Input: part model. Units: mm. Frame: model coordinates. A direction names the side the tool comes from. Round coordinates to 2 decimals unless told otherwise and drop trailing zeros. Loops run counter-clockwise (first coordinate to the right, second up) from the corner with the lowest first, then second, coordinate; pieces in that order, holes last. Notation, with made-up numbers: (-3.5, 69) - (13.5, 69) arc R28 ccw to (13.5, 93) - close; hole circle Ø3 at (-19, -1). An arc over 180 degrees is marked (long way). One line per question, with ' | ' between items. Start each with the question number.
Item 1: Section B-B, the plane z = 1.55. Return loops of the section in (x, y), plus the area to 3 significant figures.
Item 2: Material intervals for line 1 along X through (y, z) = (18.5, 1.85); line 2 along X through (y, z) = (35, 0.4); line 3 along X through (y, z) = (2.5, 2.4), sorted ascending.
Item 3: Section A-A, the plane y = 24.5. Return loops of the section in (x, z), plus the area to 3 significant figures.
Item 4: Section C-C, the plane x = -2.5. Return loops of the section in (y, z), plus the area to 3 significant figures.
Item 5: First-contact query: pin 1 (1.5 mm diameter, centred on x = -70.5, z = 1.5, fed in from +Y); pin 2 (0.9 mm diameter, centred on y = 17.5, z = 1, fed in from -X). Flat tips, straight axial feed; report the tip coordinate or a pass-through.
Item 6: Draft query along Y for faces 1 (the face through (7.729, 32.186, 1.521)), 2 (the face through (72.375, 19, 1)), 3 (the face through (-63.973, 35.741, 1.521)). Return one class per face: pulls with the +Y half, pulls with the -Y half, needs draft (parallel to the pull), parting line crosses it, or undercut.
Item 7: Set-up query: faces 4 (the face through (-71, -1.252, 1)), 5 (the face through (-71, 8.748, 1)), 6 (the face through (75.227, 1.755, 1.521)), 7 (the face through (86, 8.748, 1)), 8 (the face through (7, 29, 3)). Return all of +Z, -Z, +X, -X, +Y, -Y with unobstructed straight access to the full face (end or side cutting, diameter ignored); none if empty.
```python
from build123d import *

# Parameters (mm, degrees)
SKETCH2_R           = 1.6
BOSS_EXTRUDE1_DEPTH = 3
CUT_EXTRUDE1_REACH  = 100.01
SKETCH3_R           = 1.6
FILLET1_R           = 10
FILLET2_R           = 2


with BuildPart() as part:
    # Sketch2 → Boss-Extrude1 (new body)
    with BuildSketch(Plane.XY):
        Polygon((-74.424572317, -1.251944012), (-56.824572317, -1.251944012), (-56.824572317, 28.748055988), (72.375427683, 28.748055988), (72.375427683, -1.251944012), (89.975427683, -1.251944012), (89.975427683, 8.748055988), (82.375427683, 8.748055988), (82.375427683, 38.748055988), (-66.824572317, 38.748055988), (-66.824572317, 8.748055988), (-74.424572317, 8.748055988), align=None)
        with Locations((-70.424572317, 3.748055988)):
            Circle(SKETCH2_R, mode=Mode.SUBTRACT)
        with Locations(Location((85.975427683, 3.748055988, 0), (0, 0, 180))):
            Circle(SKETCH2_R, mode=Mode.SUBTRACT)
    extrude(amount=BOSS_EXTRUDE1_DEPTH)

    # Sketch3 → Cut-Extrude1 (cut, up to next)
    with BuildSketch(Plane.XY.offset(3), mode=Mode.PRIVATE) as cut_extrude1_sk1:
        with Locations((-36.924572317, 33.748055988)):
            Circle(SKETCH3_R)
    cut_extrude1_tool1 = extrude(cut_extrude1_sk1.sketch, amount=-CUT_EXTRUDE1_REACH, mode=Mode.PRIVATE) & part.part
    # Sketch3 → Cut-Extrude1 (cut, up to next)
    with BuildSketch(Plane.XY.offset(3), mode=Mode.PRIVATE) as cut_extrude1_sk2:
        with Locations((8.075427683, 33.748055988)):
            Circle(SKETCH3_R)
    cut_extrude1_tool2 = extrude(cut_extrude1_sk2.sketch, amount=-CUT_EXTRUDE1_REACH, mode=Mode.PRIVATE) & part.part
    # Sketch3 → Cut-Extrude1 (cut, up to next)
    with BuildSketch(Plane.XY.offset(3), mode=Mode.PRIVATE) as cut_extrude1_sk3:
        with Locations((53.075427683, 33.748055988)):
            Circle(SKETCH3_R)
    cut_extrude1_tool3 = extrude(cut_extrude1_sk3.sketch, amount=-CUT_EXTRUDE1_REACH, mode=Mode.PRIVATE) & part.part
    add(cut_extrude1_tool1.solids().sort_by_distance((-36.924572, 33.748056, 3))[0], mode=Mode.SUBTRACT)
    add(cut_extrude1_tool2.solids().sort_by_distance((8.075428, 33.748056, 3))[0], mode=Mode.SUBTRACT)
    add(cut_extrude1_tool3.solids().sort_by_distance((53.075428, 33.748056, 3))[0], mode=Mode.SUBTRACT)

    # Fillet1
    fillet1_edges = [part.edges().sort_by_distance(p)[0] for p in [
        (-66.824572317, 38.748055988, 1.5),
        (82.375427683, 38.748055988, 1.5),
        (72.375427683, -1.251944012, 1.5),
        (-56.824572317, -1.251944012, 1.5),
    ]]
    fillet(fillet1_edges, radius=FILLET1_R)

    # Fillet2
    fillet2_edges = [part.edges().sort_by_distance(p)[0] for p in [
        (-74.424572317, 8.748055988, 1.5),
        (-66.824572317, 8.748055988, 1.5),
        (82.375427683, 8.748055988, 1.5),
        (89.975427683, 8.748055988, 1.5),
    ]]
    fillet(fillet2_edges, radius=FILLET2_R)


solid = part.part
```
Return value:
1) outline: (-74.42, -1.25) - (-66.82, -1.25) arc R10 ccw to (-56.82, 8.75) - (-56.82, 28.75) - (72.38, 28.75) - (72.38, 8.75) arc R10 ccw to (82.38, -1.25) - (89.98, -1.25) - (89.98, 6.75) arc R2 ccw to (87.98, 8.75) - (84.38, 8.75) arc R2 cw to (82.38, 10.75) - (82.38, 28.75) arc R10 ccw to (72.38, 38.75) - (-56.82, 38.75) arc R10 ccw to (-66.82, 28.75) - (-66.82, 10.75) arc R2 cw to (-68.82, 8.75) - (-72.42, 8.75) arc R2 ccw to (-74.42, 6.75) - close; hole circle Ø3.2 at (-70.42, 3.75); hole circle Ø3.2 at (-36.92, 33.75); hole circle Ø3.2 at (8.08, 33.75); hole circle Ø3.2 at (53.08, 33.75); hole circle Ø3.2 at (85.98, 3.75) | area: 2,120 mm2
2) line 1: -66.82 to -56.82, 72.38 to 82.38 | line 2: -64.63 to -37.92, -35.93 to 7.08, 9.07 to 52.08, 54.07 to 80.18 | line 3: -74.42 to -71.43, -69.42 to -59.02, 74.57 to 84.97, 86.98 to 89.98
3) outline: (-66.82, 0) - (-56.82, 0) - (-56.82, 3) - (-66.82, 3) - close; (72.38, 0) - (82.38, 0) - (82.38, 3) - (72.38, 3) - close | area: 60.0 mm2
4) outline: (28.75, 0) - (38.75, 0) - (38.75, 3) - (28.75, 3) - close | area: 30.0 mm2
5) pin 1: y = 8.75 | pin 2: x = -66.82
6) face 1: undercut | face 2: needs draft | face 3: pulls with the +Y half
7) face 4: +Z, -Z, +X, -X, -Y | face 5: +Z, -Z, -X, +Y | face 6: +Z, -Z, -Y | face 7: +Z, -Z, +X, +Y | face 8: +Z, +X, -X, +Y, -Y
